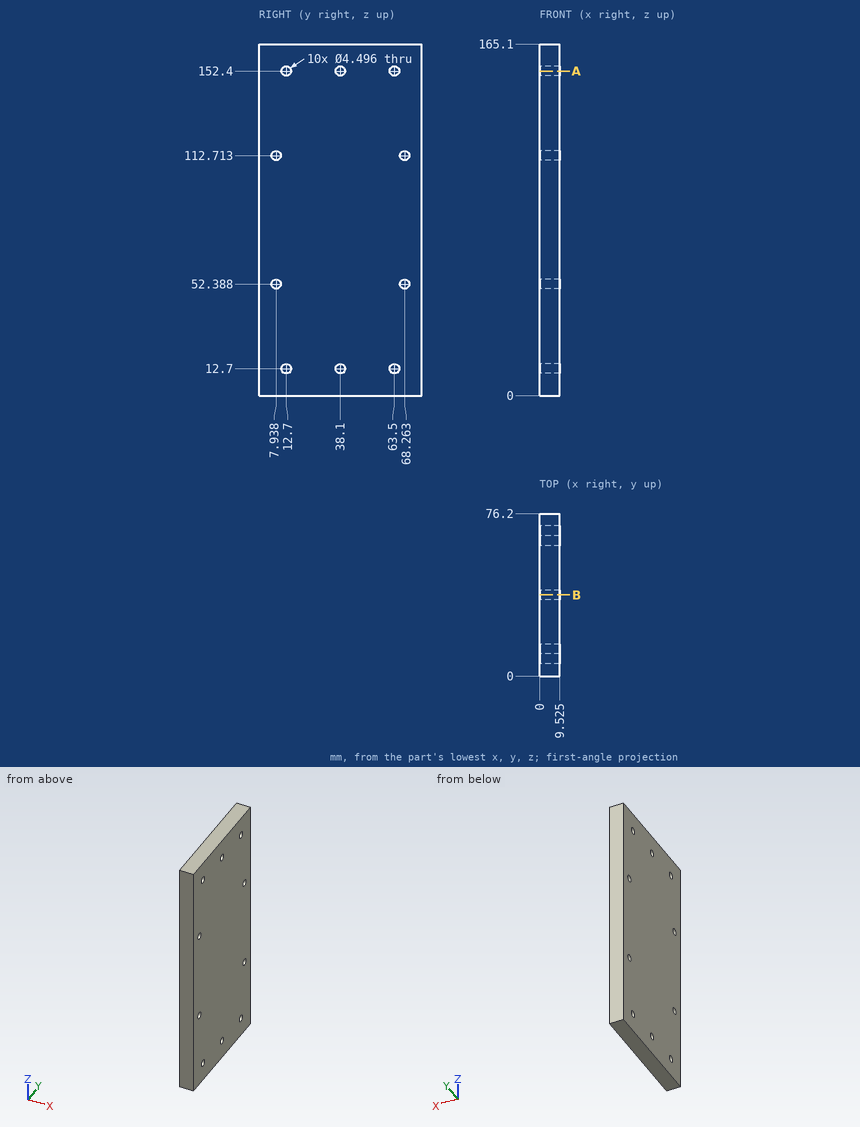
For this review, use the dimensioned drawing (mm, ordinates from the lowest corner) and the shaded views. Round coordinates to 2 decimals unless told otherwise and drop trailing zeros. Order: outer loops, then holes, each group sorted by start corner. A loop starts at its lowest first (then second) coordinate and runs counter-clockwise, first axis right, second up. Notation, with made-up numbers: (84, -12.75) -> (134, -12.75) arc R17 cw to (134, -4.75) -> close; hole circle Ø9 at (-11, 46.5). An arc over 180 degrees is marked (long way). Put each result on its own line as item: value.
Q1. For probe 1 along Y at (x, z) = (7, 12.7); probe 2 along Y at (x, z) = (3.75, 112.5) (1 decimal); probe 3 along Z at (x, y) = (3, 65.5) (1 decimal), list the stretches that pass through material, from the lowest coordinate up. Write a range as [from, to].
Check result:
probe 1: [0, 10.45], [14.95, 35.85], [40.35, 61.25], [65.75, 76.2]
probe 2: [0, 5.7], [10.2, 66], [70.5, 76.2]
probe 3: [0, 11.7], [13.7, 151.4], [153.4, 165.1]
Q2. Add section A-A on z = 152.4. Write out the cut boundary in (x, y) (1 decimal).
Check result:
outline: (0, 0) -> (9.5, 0) -> (9.5, 10.5) -> (0, 10.5) -> close; (0, 14.9) -> (9.5, 14.9) -> (9.5, 35.9) -> (0, 35.9) -> close; (0, 40.3) -> (9.5, 40.3) -> (9.5, 61.3) -> (0, 61.3) -> close; (0, 65.7) -> (9.5, 65.7) -> (9.5, 76.2) -> (0, 76.2) -> close
Q3. Add section B-B on y = 38.1. Write out the cut boundary in (x, z) (1 decimal), plus the area to 3 significant figures.
Check result:
outline: (0, 0) -> (9.5, 0) -> (9.5, 10.5) -> (0, 10.5) -> close; (0, 14.9) -> (9.5, 14.9) -> (9.5, 150.2) -> (0, 150.2) -> close; (0, 154.6) -> (9.5, 154.6) -> (9.5, 165.1) -> (0, 165.1) -> close
area: 1,490 mm2
